from build123d import *

# Parameters (mm, degrees)
SKETCH3_R               = 4.75
WIRE_HOLE_CUT_DEPTH     = 22.260291625
FRONT_STRAIN_FILLET_R   = 1
REAR_STRAIN_FILLET_R    = 1.5
SPLIT_CUT_1_DEPTH       = 22.260291625
SPLIT_CUT_2_DEPTH       = 22.26029171
WIRE_INSERT_NOTCH_DEPTH = 22.259351006


with BuildPart() as part:
    # Sketch2 → Body Revolve1 (revolve)
    with BuildSketch(Plane(origin=(0, 0, 0), x_dir=(0, 0, -1), z_dir=(1, 0, 0)), mode=Mode.PRIVATE) as body_revolve1_sk:
        Polygon((0, 0), (-18, 0), (-18, 5.51269272), (-17, 6.51269272), (0, 8), align=None)
    revolve(body_revolve1_sk.sketch.rotate(Axis((0, 0, 18), (0, 0, 1)), 90), axis=Axis((0, 0, 18), (0, 0, 1)))

    # Sketch3 → Wire Hole Cut (cut, through all)
    with BuildSketch(Plane.XY):
        Circle(SKETCH3_R)
    extrude(amount=WIRE_HOLE_CUT_DEPTH, mode=Mode.SUBTRACT)

    # Front Strain Fillet
    # the kernel refuses this fillet: 1 mm, written as the material it takes off along each edge
    with BuildSketch(Plane(origin=(0, 0, 18), x_dir=(1, 0, 0), z_dir=(0, 1, 0))) as front_strain_fillet_piece_1:
        with BuildLine():
            CenterArc((5.75, 0.971434637), FRONT_STRAIN_FILLET_R, 180, 76.272331842)
            Line((4.75, 0.971434637), (4.73, 0.971434637))
            Line((4.73, 0.971434637), (4.73, 0))
            Line((4.73, 0), (4.75, -0.02))
            ThreePointArc((4.75, -0.02), (5.13134636, -0.02), (5.507946574, -0.019428693))
            Line((5.507946574, -0.019428693), (5.51269272, 0))
        make_face()
    revolve(axis=Axis((0, 0, 18), (0, 0, -1)), mode=Mode.SUBTRACT)

    # Rear Strain Fillet
    rear_strain_fillet_edges = [part.edges().sort_by_distance(p)[0] for p in [
        (-4.75, 0, 0),
    ]]
    fillet(rear_strain_fillet_edges, radius=REAR_STRAIN_FILLET_R)

    # Sketch5 → Split Cut 1 (cut, through all)
    with BuildSketch(Plane(origin=(0, 0, 0), x_dir=(0, 0, -1), z_dir=(1, 0, 0))):
        Polygon((-18, 0), (-11.5, 0), (-11.5, 1), (-6.5, 1), (-6.5, 0), (0, 0), (0, -0.2), (-6.7, -0.2), (-6.7, 0.8), (-11.3, 0.8), (-11.3, -0.2), (-18, -0.2), align=None)
    extrude(amount=-SPLIT_CUT_1_DEPTH, mode=Mode.SUBTRACT)

    # Sketch7 → Split Cut 2 (cut, through all)
    with BuildSketch(Plane(origin=(0, 0, 0), x_dir=(0, 0, -1), z_dir=(1, 0, 0))):
        Polygon((-18, 0), (-11.5, 0), (-11.5, -1), (-6.5, -1), (-6.5, 0), (0, 0), (0, -0.2), (-6.3, -0.2), (-6.3, -1.2), (-11.7, -1.2), (-11.7, -0.2), (-18, -0.2), align=None)
    extrude(amount=SPLIT_CUT_2_DEPTH, mode=Mode.SUBTRACT)


with BuildPart() as split_cut_2_kept_piece:
    # of the separate pieces the step leaves, the one the design keeps (split_cut_2_pieces_kept)
    add(part.part.solids().sort_by_distance((6.24679918, -0.2, 0))[0])

    # Sketch6 → Wire Insert Notch (cut, through all)
    with BuildSketch(Plane.XY):
        with BuildLine():
            Line((-4.75, 0), (-4.75, 2))
            Line((-4.75, 2), (4.75, 2))
            Line((4.75, 2), (4.75, 0))
            ThreePointArc((4.75, 0), (0, -4.75), (-4.75, 0))
        make_face()
    extrude(amount=WIRE_INSERT_NOTCH_DEPTH, mode=Mode.SUBTRACT)


solid = split_cut_2_kept_piece.part
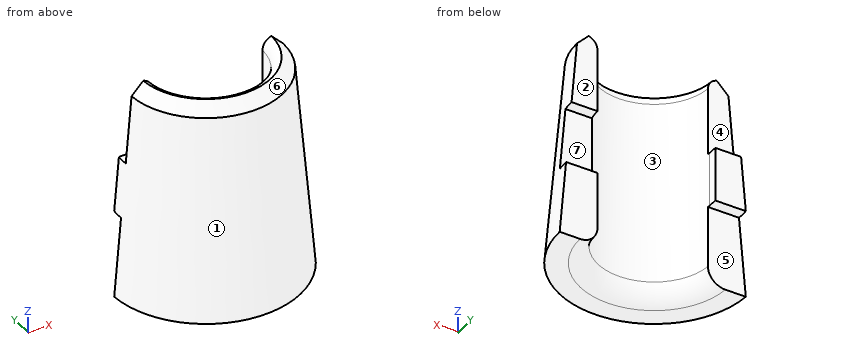
Design review of the part built by this model. Coordinates are the model's own, in mm. Face numbers are marked on the shaded views. A direction names the side the tool comes from. Round coordinates to 2 decimals unless told otherwise and drop trailing zeros. Write each loop counter-clockwise with the first axis right and the second up, starting at its lowest first coordinate (ties: lowest second). Pieces come first, ordered by that corner, then holes. Notation, with made-up numbers: M 70,53 L 89,53 A21 cw 89,78 Z; hole C 75,-20 d7. An arc over 180 degrees is marked long. One line per item, written item: value. Start each with the question number.
1. Take a section at A-A on x = 0. State the section outline as (y, z) points.
2. Draft analysis for pull direction X (two halves, no side actions). For the marked faces 1, 2 and 3, state which applies: pulls with the +X half, pulls with the -X half, needs draft (parallel to the pull), parting line crosses it, or undercut.
3. Take a section at C-C on y = -0.5. State how many separate pieces and enclosed holes the cut face has, then the cut area to 3 significant figures.
4. Clearance check with flat-ended pins moving along their axes: P1, Ø2, axis at x = 6, z = 8, coming from the +Y side; P2, Ø1.8, axis at x = -5.5, z = 13.5, coming from the +Y side; P3, Ø0.8, axis at x = -5.5, y = 0, coming from the -Z side. State where each tip first meets the part, or that it passes through.
5. For the marked faces 4, 5, 6 and 7, list the 3-axis set-ups (+Z, -Z, +X, -X, +Y, -Y) from which the entire face can be reached by the end or side of a thin tool; tool diameter is ignored.
6. To check wall thickness, follow probe 1 along X at (y, z) = (-1.75, 14.5); probe 2 along X at (y, z) = (-2.25, 12.25); probe 3 along Y at (x, z) = (5.25, 16.25). State the ranges of each line that lie inside material, in increasing order. Write a range as from..to.
Computed:
1. outline: M -8,0 L -6.25,0 A1.5 ccw -4.75,1.5 L -4.75,17.03 A1 ccw -5.51,18 L -6.51,17 Z
2. face 1: parting line crosses it
2. face 2: needs draft
2. face 3: undercut
3. separate pieces: 3
3. enclosed holes: 0
3. area: 73.4 mm²
4. P1: stops at y = -1.2
4. P2: stops at y = -0.2
4. P3: stops at z = 0.05
5. face 4: +Z, +X, -X, +Y
5. face 5: -Z, +X, -X, +Y
5. face 6: +Z, -Y
5. face 7: +X, +Y
6. probe 1: x = -6.5..-4.42, 4.42..6.5
6. probe 2: x = -6.55..-4.18, 4.18..6.55
6. probe 3: y = -3.96..-0.2
